from build123d import *

# Parameters (mm, degrees)
SKETCH1_W           = 44
SKETCH1_H           = 24
BOSS_EXTRUDE1_DEPTH = 1.9
FILLET1_R           = 1


with BuildPart() as part:
    # Sketch1 → Boss-Extrude1 (new body)
    with BuildSketch(Plane(origin=(0, 0, 0), x_dir=(1, 0, 0), z_dir=(0, 1, 0))):
        Rectangle(SKETCH1_W, SKETCH1_H)
    extrude(amount=BOSS_EXTRUDE1_DEPTH)

    # Loft2: read off the stored shape, not the designer's step
    # Loft2: loft between two sections, ruled curve by curve
    loft2_from = [
        Edge.make_bspline([(-13.96783709, 7.9, 3.975674545), (-21.919186181, 7.9, 10.040000365), (-27.983512, 7.9, 2.088651274), (-20.03216291, 7.9, -3.975674545), (-12.080813819, 7.9, -10.040000365), (-6.016488, 7.9, -2.088651274), (-13.96783709, 7.9, 3.975674545)], [0, 0, 0, 0, 0.5, 0.5, 0.5, 1, 1, 1, 1], 3, [1, 0.333333333, 0.333333333, 1, 0.333333333, 0.333333333, 1]),
    ]
    loft2_to = [
        Edge.make_bspline([(-14.73827925, 1.9, -1.065185077), (-12.607909097, 1.9, 3.458256424), (-17.131350597, 1.9, 5.588626577), (-19.26172075, 1.9, 1.065185077), (-21.392090903, 1.9, -3.458256424), (-16.868649403, 1.9, -5.588626577), (-14.73827925, 1.9, -1.065185077)], [0, 0, 0, 0, 0.5, 0.5, 0.5, 1, 1, 1, 1], 3, [1, 0.333333333, 0.333333333, 1, 0.333333333, 0.333333333, 1]),
    ]
    loft2 = Solid(Shell([*[Face.make_surface_from_curves(loft2_from[k], loft2_to[k]) for k in range(1)], Face(Wire(loft2_from)), Face(Wire(loft2_to))]))
    add(loft2)

    # Fillet1
    fillet1_edges = [part.edges().sort_by_distance(p)[0] for p in [
        (-20.03216291, 7.9, -3.975674545),
    ]]
    fillet(fillet1_edges, radius=FILLET1_R)


solid = part.part
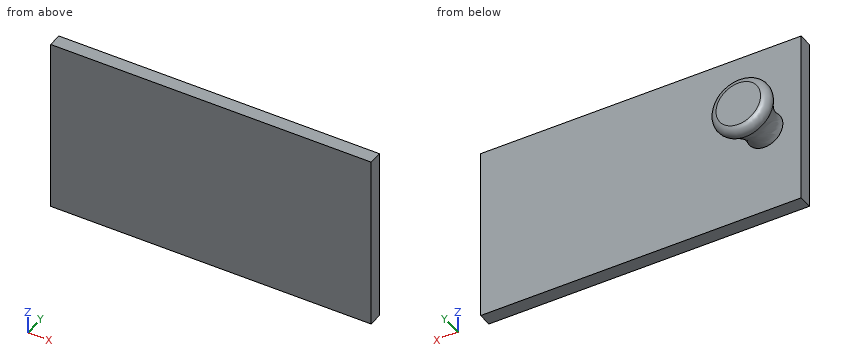
Here's how the part is built. I have some questions about the finished solid (model axes, mm). Round coordinates to 2 decimals unless told otherwise and drop trailing zeros. Order: outer loops, then holes, each group sorted by start corner. A loop starts at its lowest first (then second) coordinate and runs counter-clockwise, first axis right, second up. Notation, with made-up numbers: M -11,-13.5 L 2,-13.5 A36 ccw 2,21.5 Z; hole C 23,55.5 d4. An arc over 180 degrees is marked long. One line per question, with ' | ' between items.
1) Imagine slicing it at B-B, the plane x = 15.5. Write out the boundary of the cut face in (y, z).
Checked values:
outline: M 0,-12 L 1.9,-12 L 1.9,12 L 0,12 Z
2) Imagine slicing it at A-A, the plane z = -7.5. Write out the boundary of the cut face in (x, y), plus the area to 3 significant figures.
Checked values:
outline: M -22,0 L 22,0 L 22,1.9 L -22,1.9 Z | area: 83.6 mm²
3) I'm going to push flat-ended pins straight in: pin 1 Ø2 at (x, z) = (-6, -3.5) entering from +Y; pin 2 Ø12 at (x, z) = (-15, 9.5) entering from +Y. Where does each tip first touch, or does it pass through?
Checked values:
pin 1: stops at y = 1.9 | pin 2: stops at y = 7.66
4) I need wall thicknesses on line 1 (Y direction, x = -11, z = 1.75); line 2 (X direction, y = 7.5, z = -0.25); line 3 (X direction, y = 5, z = -1.5). Which ranges of each line are inside material? Lowest first, please.
Checked values:
line 1: y = 0 to 1.9 | line 2: x = -20.85 to -13.15 | line 3: x = -19.68 to -14.32
